from build123d import *

# Parameters (mm, degrees)
SKETCH_1_R      = 1.6
EXTRUDE_7_DEPTH = 2.8
EXTRUDE_8_DEPTH = 0.5
EXTRUDE_9_DEPTH = 4.3


with BuildPart() as part:
    # Sketch 1 → Extrude 7 (new body)
    with BuildSketch(Plane.XY):
        Polygon((22.5, -30.5), (22.5, 19.601020514), (27.5, 24.5), (27.5, 30.5), (-22.5, 30.5), (-22.5, -30.5), align=None)
        Polygon((21, -29), (-20.5, -29), (-20.5, 29), (-18, 29), (-18, 26), (9, 26), (9, 27.5), (21, 27.5), (21, -9.279002621), (16, -9.279002621), (16, -13), (4, -13), (4, -18), (21, -18), align=None, mode=Mode.SUBTRACT)
        with Locations((25, 27.5)):
            Circle(SKETCH_1_R, mode=Mode.SUBTRACT)
    extrude(amount=-EXTRUDE_7_DEPTH)

    # Sketch 1_11 → Extrude 8 (add)
    with BuildSketch(Plane.XY):
        Polygon((16, -9.279002621), (21, -9.279002621), (21, 12), (-18, 12), (-18, -6), (-8, -6), (-8, -18), (4, -18), (4, -6), (16, -6), align=None)
    extrude(amount=-EXTRUDE_8_DEPTH)

    # Sketch 1_12 → Extrude 9 (add)
    with BuildSketch(Plane.XY):
        Polygon((-20.5, -29), (21, -29), (21, -18), (16, -18), (4, -18), (-2, -18), (-8, -18), (-18, -18), (-18, -6), (-18, 12), (-18, 26), (-18, 27.5), (-18, 29), (-20.5, 29), align=None)
    extrude(amount=-EXTRUDE_9_DEPTH)


solid = part.part
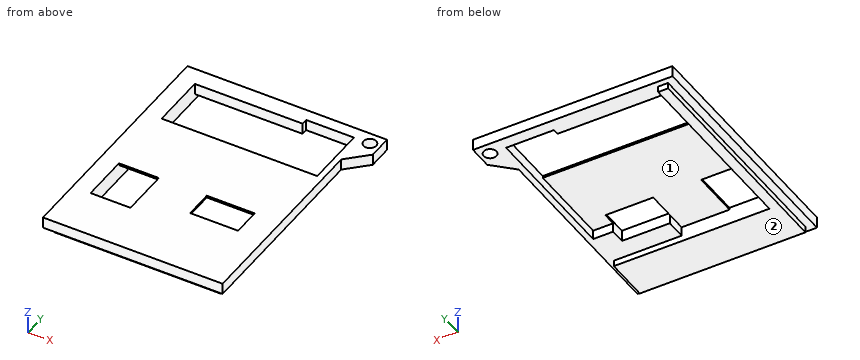
Work out the finished part from the listing and answer in its coordinate system (mm). Face numbers are marked on the shaded views. Round coordinates to 2 decimals unless told otherwise and drop trailing zeros. Write each loop counter-clockwise with the first axis right and the second up, starting at its lowest first coordinate (ties: lowest second). Pieces come first, ordered by that corner, then holes. Notation, with made-up numbers: (25.5, -23.75) -> (45.5, -23.75) arc R14 cw to (45.5, -6.75) -> close; hole circle Ø7 at (12, -26). An arc over 180 degrees is marked (long way). Answer as CSV lines item,"result". Start each with the question number.
(1) Find the intervals of material crossed by probe 1 along X at (y, z) = (-11, -1.85); probe 2 along X at (y, z) = (-5, -0.85); probe 3 along Y at (x, z) = (-9.5, -2.45), in increasing order.
(2) The part is cut by section D-D, the plane x = -14. Give the vertices of the cut face in (y, z).
(3) The part is cut by section B-B, the plane x = 20. Give the vertices of the cut face in (y, z), then the cut area to 3 significant figures.
(4) The mould has two halves that part along Y. Classify the marked faces 1 and 2: +Y half, -Y half, draft (parallel to the pull), parting line (faces both ways), or undercut.
(5) Each of these flat-tipped pins is pushed along its axis until it touches: pin 1 (0.8 mm diameter, centred on y = -25.5, z = -3.5, fed in from +X); pin 2 (1 mm diameter, centred on x = -11.5, y = 6, fed in from -Z); pin 3 (1.6 mm diameter, centred on y = 2, z = -4, fed in from -X). Where does it stop, or does it pass through?
(6) The part is cut by section C-C, the plane z = -1.75. Give the vertices of the cut face in (x, y), then the cut area to 3 significant figures.
(7) The part is cut by section A-A, the plane y = -7.5. Give the vertices of the cut face in (x, z), then the cut area to 4 significant figures.
Output values:
1,probe 1,"x = -22.5 to -18, 16 to 22.5"
1,probe 2,"x = -22.5 to -18, 21 to 22.5"
1,probe 3,"y = -30.5 to -18, 26 to 30.5"
2,outline,"(-30.5, -2.8) -> (-29, -2.8) -> (-29, -4.3) -> (-18, -4.3) -> (-18, 0) -> (-30.5, 0) -> close; (-6, -0.5) -> (12, -0.5) -> (12, 0) -> (-6, 0) -> close; (26, -2.8) -> (30.5, -2.8) -> (30.5, 0) -> (26, 0) -> close"
3,outline,"(-30.5, -2.8) -> (-29, -2.8) -> (-29, -4.3) -> (-18, -4.3) -> (-18, -2.8) -> (-9.28, -2.8) -> (-9.28, -0.5) -> (12, -0.5) -> (12, 0) -> (-30.5, 0) -> close; (27.5, -2.8) -> (30.5, -2.8) -> (30.5, 0) -> (27.5, 0) -> close"
3,area,"95.0 mm²"
4,face 1,"undercut"
4,face 2,"draft"
5,pin 1,"stops at x = 21"
5,pin 2,"stops at z = -0.5"
5,pin 3,"stops at x = -20.5"
6,outline,"(-22.5, -30.5) -> (22.5, -30.5) -> (22.5, 19.6) -> (27.5, 24.5) -> (27.5, 30.5) -> (-22.5, 30.5) -> close; hole (-18, -18) -> (4, -18) -> (4, -13) -> (16, -13) -> (16, -9.28) -> (21, -9.28) -> (21, 27.5) -> (9, 27.5) -> (9, 26) -> (-18, 26) -> close; hole circle Ø3.2 at (25, 27.5)"
6,area,"1,150 mm²"
7,outline,"(-22.5, -2.8) -> (-20.5, -2.8) -> (-20.5, -4.3) -> (-18, -4.3) -> (-18, 0) -> (-22.5, 0) -> close; (-8, -0.5) -> (4, -0.5) -> (4, 0) -> (-8, 0) -> close; (16, -0.5) -> (21, -0.5) -> (21, -2.8) -> (22.5, -2.8) -> (22.5, 0) -> (16, 0) -> close"
7,area,"29.05 mm²"
